```python
from build123d import *

# Parameters (mm, degrees)
F1_DEPTH       = 3
F2_R           = 4.99999
F4_D           = 2.4384
F4_CBORE_D     = 5.2
F4_CBORE_DEPTH = 1.5
F5_W           = 30
F5_H           = 25
F6_DEPTH       = 12
F8_DEPTH       = 25.001
F9_T1_DEPTH    = 66.0035618315
F10_SIZE       = 4


# Not quite as in the source:
# - a fillet or chamfer that OpenCascade refuses, or shapes differently, is made with other operations: its cross-section is extruded or revolved along the edge and cut away or added
# - a fillet or chamfer is up to 0.001 mm smaller than in the source, because OpenCascade refuses the exact size


with BuildPart() as f1:
    # F0 (on Top) → F1 (new body)
    with BuildSketch(Plane.XY):
        with BuildLine():
            ThreePointArc((18.0125, 0), (0, -18.0125), (-18.0125, 0))
            Line((-18.0125, 0), (-18.0125, 5))
            Line((-18.0125, 5), (-28.0125, 5))
            Line((-28.0125, 5), (-28.0125, 0))
            ThreePointArc((-28.0125, 0), (0, -28.0125), (28.0125, 0))
            Line((28.0125, 0), (28.0125, 5))
            Line((28.0125, 5), (18.0125, 5))
            Line((18.0125, 5), (18.0125, 0))
        make_face()
    extrude(amount=F1_DEPTH)

    # F2 (radius 5 in the source; OpenCascade refuses exactly that, so slightly less here)
    f2_edges = [f1.edges().sort_by_distance(p)[0] for p in [
        (-28.0125, 5, 1.5),
        (-18.0125, 5, 1.5),
        (18.0125, 5, 1.5),
        (28.0125, 5, 1.5),
    ]]
    fillet(f2_edges, radius=F2_R)

    # F4 (through all)
    with Locations(Plane.XY.offset(3)):
        with Locations((-23.0125, 0), (23.0125, 0)):
            CounterBoreHole(F4_D / 2, F4_CBORE_D / 2, F4_CBORE_DEPTH)

    # F5 (on Top) → F6 (join)
    with BuildSketch(Plane.XY):
        with Locations((0, -30.5125)):
            Rectangle(F5_W, F5_H)
    extrude(amount=F6_DEPTH)

    # F7 (on face) → F8 (cut, through all)
    with BuildSketch(Plane(origin=(0, -18.0125, 0), x_dir=(-1, 0, 0), z_dir=(0, 1, 0))):
        Polygon((0, 3), (10.1, 3), (10.1, 9.7), (-10.1, 9.7), (-10.1, 3), align=None)
    extrude(amount=-F8_DEPTH, mode=Mode.SUBTRACT)

    # F9: chamfer of 7 on 1 edges, made by hand

    # F9_s2 → F9_t1 (cut)
    with BuildSketch(Plane.YZ.offset(-33.0017809158)):
        Polygon((-25.0125, 12), (-18.0125, 5), (-18.0125, 12), align=None)
    extrude(amount=F9_T1_DEPTH, mode=Mode.SUBTRACT)

    # F10
    f10_edges = [f1.edges().sort_by_distance(p)[0] for p in [
        (-15, -43.0125, 6),
        (15, -43.0125, 6),
    ]]
    chamfer(f10_edges, length=F10_SIZE)


solid = f1.part
```
Here's how the part is built. I have some questions about the finished solid (model axes, mm). A direction names the side the tool comes from. Round coordinates to 2 decimals unless told otherwise and drop trailing zeros. Order: outer loops, then holes, each group sorted by start corner. A loop starts at its lowest first (then second) coordinate and runs counter-clockwise, first axis right, second up. Notation, with made-up numbers: M -3,-34 L 51,-34 A8 cw 51,-23 Z; hole C 37.5,52.25 d7. An arc over 180 degrees is marked long. One line per question, with ' | ' between items.
1) I want a section at A-A, the plane y = -37. Write out the boundary of the cut face in (x, z).
Working result:
outline: M -15,0 L 15,0 L 15,12 L -15,12 Z; hole M -10.1,3 L 10.1,3 L 10.1,9.7 L -10.1,9.7 Z
2) For pin 1 Ø1.6 at (x, y) = (23.5, 0.5) entering from +Z; pin 2 Ø1.6 at (x, z) = (-13.5, 4) entering from +Y; pin 3 Ø6 at (y, z) = (-30, 9) entering from +X; pin 4 Ø2 at (x, y) = (23.01, 0) entering from -Z, each with a flat end and sliding along its axis, tell me the tip position at first contact or that it passes through.
Working result:
pin 1: z = 1.5 | pin 2: y = -18.01 | pin 3: x = 15 | pin 4: through
3) I want a section at D-D, the plane x = -14. Write out the boundary of the cut face in (y, z), then the cut area to 3 significant figures.
Working result:
outline: M -40.01,0 L -11.33,0 L -11.33,3 L -18.01,3 L -18.01,5 L -25.01,12 L -40.01,12 Z | area: 260 mm²
4) I need wall thicknesses on line 1 along Z through (x, y) = (6.5, -34); line 2 along Z through (x, y) = (-9, -23.5); line 3 along Z through (x, y) = (25, -1). Which ranges of each line are inside material? Lowest first, please.
Working result:
line 1: 0 to 3, 9.7 to 12 | line 2: 0 to 3, 9.7 to 10.49 | line 3: 0 to 1.5
5) I want a section at B-B, the plane x = 0. Write out the boundary of the cut face in (y, z), then the cut area to 3 significant figures.
Working result:
outline: M -43.01,0 L -18.01,0 L -18.01,3 L -43.01,3 Z; M -43.01,9.7 L -22.71,9.7 L -25.01,12 L -43.01,12 Z | area: 119 mm²
6) For faces 5 (the face through (25.492, 0.781, 2.26)), 6 (the face through (-19.44, 3.5, 1.52)), 7 (the face through (-10.1, -30, 6)), which set-ups out of +Z, -Z, +X, -X, +Y, -Y let a thin tool reach every point of the face, with its end or its side?
Working result:
face 5: +Z | face 6: +Z, -Z, +Y | face 7: +Y, -Y
7) If we mould it in two halves opening along Z, with no side actions, what happens to faces 1 (the face through (0, -19, 3)), 2 (the face through (26.587, 3.496, 1.521)), 3 (the face through (10.1, -30, 6)), 4 (the face through (24, -1, 1.5))? For each: +Z half, -Z half, draft (parallel to the pull), parting line (faces both ways), or undercut.
Working result:
face 1: undercut | face 2: draft | face 3: undercut | face 4: +Z half
8) I want a section at C-C, the plane z = 9. Write out the boundary of the cut face in (x, y).
Working result:
outline: M -15,-39.01 L -11,-43.01 L -10.1,-43.01 L -10.1,-22.01 L -15,-22.01 Z; M 10.1,-43.01 L 11,-43.01 L 15,-39.01 L 15,-22.01 L 10.1,-22.01 Z
